Autodesk Inventor part; units mm, degrees
ref_plane "YZ Plane" through (0, 0, 0) normal (1, 0, 0) x (0, 1, 0)
ref_plane "XZ Plane" through (0, 0, 0) normal (0, 1, 0) x (-1, 0, 0)
ref_plane "XY Plane" through (0, 0, 0) normal (0, 0, 1) x (1, 0, 0)
sketch "Sketch1" plane through (0, 0, 0) normal (0, 0, 1) x (1, 0, 0)
  line L0 (0, 0) -> (23.8603, 3.5978)
  line L1 (23.8603, 3.5978) -> (35.2216, -71.7505)
  line L2 (35.2216, -71.7505) -> (11.3613, -75.3483)
  line L3 (11.3613, -75.3483) -> (0, 0)
  line L4 (12.1195, 0.5431) -> (15.8869, 1.1111)
  line L5 (15.8869, 1.1111) -> (16.1899, -0.8981)
  line L6 (16.1899, -0.8981) -> (8.6551, -2.0343)
  line L7 (8.6551, -2.0343) -> (8.3521, -0.025)
  line L8 (8.3521, -0.025) -> (12.1195, 0.5431)
  line L9 (23.1021, -72.2936) -> (26.8695, -71.7255)
  line L10 (26.8695, -71.7255) -> (26.5666, -69.7162)
  line L11 (26.5666, -69.7162) -> (19.0317, -70.8524)
  line L12 (19.0317, -70.8524) -> (19.3347, -72.8616)
  line L13 (19.3347, -72.8616) -> (23.1021, -72.2936)
  dimension "d0" = 24.13
  dimension "d1" = 76.2
  dimension "d9" = 2.032
  dimension "d10" = 7.62
extrude "Extrusion1" add sketch "Sketch1" along normal blind 12.7 contours L0 L1 L2 L3 | L4 L5 L6 L7 L8 | L13 L12 L11 L10 L9
shell "Shell1" thickness 0.635 removed faces 1 at (23.4811, -47.8337, 12.7)
sketch "Sketch2" plane through (11.8946, -74.6257, 0.635) normal (0, 0, 1) x (0.9888, 0.1491, 0)
  point P0 (-0.635, 75.565)
extrude "Extrusion2" add sketch "Sketch1" along normal blind 2.54 contours L4 L5 L6 L7 L8 | L13 L12 L11 L10 L9
properties part number "batteryHousing"
Work out the finished part from the listing and answer in its coordinate system (mm). A direction names the side the tool comes from. Round coordinates to 2 decimals unless told otherwise and drop trailing zeros. Order: outer loops, then holes, each group sorted by start corner. A loop starts at its lowest first (then second) coordinate and runs counter-clockwise, first axis right, second up.
Q1. Given pin 1 Ø0.9 at (x, y) = (12, -0.5) entering from +Z; pin 2 Ø1.5 at (y, z) = (-31.5, 2.5) entering from +X; pin 3 Ø6 at (y, z) = (-53, 7) entering from -X, each flat-ended and moving along its own axis, determine where each tip first touches the part or whether it passes through.
Solution:
pin 1: stops at z = 2.54
pin 2: stops at x = 29.27
pin 3: stops at x = 7.54
Q2. A tool of negligible diameter and unlimited length cuts with its end or side. For faces 1 (the flat face through (29, -33, 12.7)), 2 (the flat face through (26.72, -70.73, 1.57)), from which of +Z, -Z, +X, -X, +Y, -Y can it reach the whole face along a straight path? Write none if from no direction.
Solution:
face 1: +Z, +X, -X, +Y, -Y
face 2: +Z
Q3. Find the intervals of material crossed by line 1 along Z through (x, y) = (12, -32) (3 decimals); line 2 along Y through (x, z) = (13, 10.5); line 3 along X through (y, z) = (-55, 9), in increasing order.
Solution:
line 1: z = 0 to 0.635
line 2: y = -75.1 to -74.46, 1.32 to 1.96
line 3: x = 8.29 to 8.94, 32.05 to 32.7
Q4. A cutting plane is placed at C-C, the plane y = -50. Determine the outline of the cut face in (x, z) (3 decimals).
Solution:
outline: (7.539, 0) - (31.942, 0) - (31.942, 12.7) - (31.3, 12.7) - (31.3, 0.635) - (8.181, 0.635) - (8.181, 12.7) - (7.539, 12.7) - close
Q5. A cutting plane is placed at B-B, the plane x = 3. Determine the outline of the cut face in (y, z) (3 decimals), then the cut area to 3 significant figures.
Solution:
outline: (-19.896, 0) - (0.452, 0) - (0.452, 12.7) - (-0.19, 12.7) - (-0.19, 0.635) - (-15.637, 0.635) - (-15.637, 12.7) - (-19.896, 12.7) - close
area: 72.1 mm2
Q6. A cutting plane is placed at A-A, the plane z = 3.25. Determine the outline of the cut face in (x, y).
Solution:
outline: (0, 0) - (11.36, -75.35) - (35.22, -71.75) - (23.86, 3.6) - close; hole (0.72, -0.53) - (11.89, -74.63) - (34.5, -71.22) - (23.33, 2.88) - close
Q7. The mould has two halves that part along Y. Classify faces 3 (the flat face through (23.458, -73.524, 6.261)), 4 (the flat face through (23.355, -72.898, 6.583)), 5 (the flat face through (17, -35, 0)), 6 (the flat face through (29.46, -33.55, 6.26)): pulls with the +Y half, pulls with the -Y half, needs draft (parallel to the pull), parting line crosses it, or undercut.
Solution:
face 3: pulls with the -Y half
face 4: undercut
face 5: needs draft
face 6: pulls with the +Y half
